```python
from build123d import *

# Parameters (mm, degrees)
ESQUISSE2_R        = 4.25
BOSS_EXTRU_1_DEPTH = 5
CONG_1_R           = 5
CONG_2_R           = 2


with BuildPart() as part:
    # Esquisse2 → Boss.-Extru.1 (new body)
    with BuildSketch(Plane.XY):
        with BuildLine():
            Line((-41.632526167, 33.200832294), (-33.836607647, 42.976604913))
            Line((-33.836607647, 42.976604913), (-40.054629461, 50.874248484))
            Line((-40.054629461, 50.874248484), (-41.75579133, 53.034930852))
            ThreePointArc((-41.75579133, 53.034930852), (-52.772575719, 42.086877432), (-60.995330499, 28.91054578))
            Line((-60.995330499, 28.91054578), (-49.426698361, 23.427249496))
            Line((-49.426698361, 23.427249496), (-41.632526167, 33.200832294))
        make_face()
        with Locations((-47.300804689, 37.721133012)):
            Circle(ESQUISSE2_R, mode=Mode.SUBTRACT)
        with BuildLine():
            Line((-41.75579133, 53.034930852), (-40.054629461, 50.874248484))
            ThreePointArc((-40.054629461, 50.874248484), (-28.093972108, 58.337734197), (-14.801436125, 63.035545438))
            Line((-14.801436125, 63.035545438), (-15.430068548, 65.712730765))
            ThreePointArc((-15.430068548, 65.712730765), (-29.28715239, 60.815398583), (-41.75579133, 53.034930852))
        make_face()
        with BuildLine():
            Line((-14.801436125, 63.035545438), (-12.503682933, 53.25))
            Line((-12.503682933, 53.25), (0, 53.25))
            Line((0, 53.25), (12.503682933, 53.25))
            Line((12.503682933, 53.25), (14.801436125, 63.035545438))
            Line((14.801436125, 63.035545438), (15.430068548, 65.712730765))
            ThreePointArc((15.430068548, 65.712730765), (0, 67.5), (-15.430068548, 65.712730765))
            Line((-15.430068548, 65.712730765), (-14.801436125, 63.035545438))
        make_face()
        with Locations((0, 60.5)):
            Circle(ESQUISSE2_R, mode=Mode.SUBTRACT)
        with BuildLine():
            Line((15.430068548, 65.712730765), (14.801436125, 63.035545438))
            ThreePointArc((14.801436125, 63.035545438), (28.093972108, 58.337734197), (40.054629461, 50.874248484))
            Line((40.054629461, 50.874248484), (41.75579133, 53.034930852))
            ThreePointArc((41.75579133, 53.034930852), (29.28715239, 60.815398583), (15.430068548, 65.712730765))
        make_face()
        with BuildLine():
            Line((41.75579133, 53.034930852), (40.054629461, 50.874248484))
            Line((40.054629461, 50.874248484), (33.836607647, 42.976604913))
            Line((33.836607647, 42.976604913), (41.632526363, 33.200832047))
            Line((41.632526363, 33.200832047), (49.426698361, 23.427249496))
            Line((49.426698361, 23.427249496), (60.995330499, 28.91054578))
            ThreePointArc((60.995330499, 28.91054578), (52.772575719, 42.086877432), (41.75579133, 53.034930852))
        make_face()
        with Locations((47.300804689, 37.721133012)):
            Circle(ESQUISSE2_R, mode=Mode.SUBTRACT)
    extrude(amount=BOSS_EXTRU_1_DEPTH)

    # Congé1
    cong_1_edges = [part.edges().sort_by_distance(p)[0] for p in [
        (60.995330499, 28.91054578, 2.5),
        (40.054629461, 50.874248484, 2.5),
        (14.801436125, 63.035545438, 2.5),
        (-14.801436125, 63.035545438, 2.5),
        (-40.054629461, 50.874248484, 2.5),
        (-60.995330499, 28.91054578, 2.5),
    ]]
    fillet(cong_1_edges, radius=CONG_1_R)

    # Congé2
    cong_2_edges = [part.edges().sort_by_distance(p)[0] for p in [
        (49.426698361, 23.427249496, 2.5),
        (33.836607647, 42.976604913, 2.5),
        (12.503682933, 53.25, 2.5),
        (-12.503682933, 53.25, 2.5),
        (-33.836607647, 42.976604913, 2.5),
        (-49.426698361, 23.427249496, 2.5),
    ]]
    fillet(cong_2_edges, radius=CONG_2_R)


solid = part.part
```
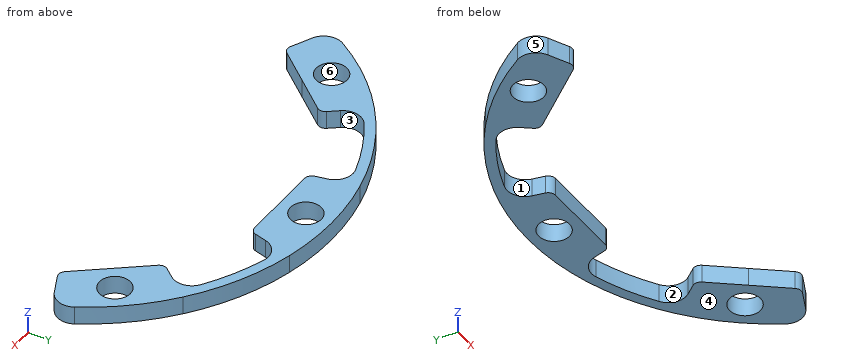
Here's how the part is built. I have some questions about the finished solid (model axes, mm). Face numbers are marked on the shaded views. A direction names the side the tool comes from. Coordinates: 2 decimals unless noted, no trailing zeros. Write each loop counter-clockwise with the first axis right and the second up, starting at its lowest first coordinate (ties: lowest second). Pieces come first, ordered by that corner, then holes. Notation, with made-up numbers: M 67,78 L 113,78 A19 ccw 113,111 Z; hole C -3.5,61 d1. An arc over 180 degrees is marked long. Answer as CSV lines item,"result". Start each with the question number.
Q1. I need wall thicknesses on probe 1 along X at (y, z) = (37, 3.35); probe 2 along X at (y, z) = (36.5, 2.9); probe 3 along X at (y, z) = (55.5, 0.9). Which ranges of each line are inside material? Lowest first, please. Write a range as [from, to].
Q2. Suppose I cut it at B-B, the plane y = 49.5. List the corners of the cut face in (x, z) for me, then the cut area to 3 significant figures.
Q3. Will these pins go through, and if not, where does the flat tip stop? pin 1 Ø3 at (x, z) = (26, 3) entering from -Y; pin 2 Ø8 at (x, y) = (-30.5, 34.5) entering from +Z; pin 3 Ø1.5 at (y, z) = (53, 3.5) entering from -X; pin 4 Ø1.5 at (x, z) = (-3.5, 2.5) entering from -Y.
Q4. Suppose I cut it at D-D, the plane z = 1.4. List the corners of the cut face in (x, y) for me, then the cut area to 3 significant figures.
Q5. For the marked faces 1 and 2, which set-ups out of +Z, -Z, +X, -X, +Y, -Y let a thin tool reach every point of the face, with its end or its side?
Q6. If we mould it in two halves opening along X, with no side actions, what happens to the marked faces 3, 4, 5 and 6? For each: pulls with the +X half, pulls with the -X half, needs draft (parallel to the pull), parting line crosses it, or undercut.
Q7. Suppose I cut it at C-C, the plane y = 60.5. List the corners of the cut face in (x, z) for me, then the cut area to 3 significant figures.
Q8. Suppose I cut it at A-A, the plane x = 0. List the corners of the cut face in (y, z) for me, then the cut area to 4 significant figures.
Entries:
1,probe 1,"x = [-56.46, -51.49], [-43.11, -38.6], [38.6, 43.11], [51.49, 56.46]"
1,probe 2,"x = [-56.78, -51.37], [-43.23, -39], [39, 43.23], [51.37, 56.78]"
1,probe 3,"x = [-38.42, -33.35], [-13.03, 13.03], [33.35, 38.42]"
2,outline,"M -45.89,0 L -37.89,0 L -37.89,5 L -45.89,5 Z; M 37.89,0 L 45.89,0 L 45.89,5 L 37.89,5 Z"
2,area,"80.0 mm²"
3,pin 1,"stops at y = 58.62"
3,pin 2,"passes through"
3,pin 3,"stops at x = -42.73"
3,pin 4,"stops at y = 53.25"
4,outline,"M -58.49,33.7 A5 ccw -56.3,26.68 L -50.86,24.11 A2 ccw -48.44,24.67 L -34.82,41.74 A2 ccw -34.82,44.22 L -36.83,46.78 A5 cw -35.66,54.05 A64.75 cw -20.02,61.58 A5 cw -13.61,57.96 L -12.87,54.79 A2 ccw -10.92,53.25 L 10.92,53.25 A2 ccw 12.87,54.79 L 13.61,57.96 A5 cw 20.02,61.58 A64.75 cw 35.66,54.05 A5 cw 36.83,46.78 L 34.82,44.22 A2 ccw 34.82,41.74 L 48.44,24.67 A2 ccw 50.86,24.11 L 56.3,26.68 A5 ccw 58.49,33.7 A67.5 ccw Z; hole C -47.3,37.72 d8.5; hole C 0,60.5 d8.5; hole C 47.3,37.72 d8.5"
4,area,"1,150 mm²"
5,face 1,"+Z, -Z, -Y"
5,face 2,"+Z, -Z"
6,face 3,"undercut"
6,face 4,"needs draft"
6,face 5,"pulls with the -X half"
6,face 6,"undercut"
7,outline,"M -29.93,0 L -23.07,0 L -23.07,5 L -29.93,5 Z; M -15.09,0 L -4.25,0 L -4.25,5 L -15.09,5 Z; M 4.25,0 L 15.09,0 L 15.09,5 L 4.25,5 Z; M 23.07,0 L 29.93,0 L 29.93,5 L 23.07,5 Z"
7,area,"177 mm²"
8,outline,"M 53.25,0 L 56.25,0 L 56.25,5 L 53.25,5 Z; M 64.75,0 L 67.5,0 L 67.5,5 L 64.75,5 Z"
8,area,"28.75 mm²"
